The listing builds one solid part. Answer for the finished solid, in the listing's coordinates (mm). Coordinates: 2 decimals unless noted, no trailing zeros. Write each loop counter-clockwise with the first axis right and the second up, starting at its lowest first coordinate (ties: lowest second). Pieces come first, ordered by that corner, then holes. Notation, with made-up numbers: M 83,-12.5 L 112,-12.5 A24 ccw 112,0.5 Z; hole C -15,61 d8. An arc over 180 degrees is marked long. Answer as CSV lines item,"result".
```python
from build123d import *

# Parameters (mm, degrees)
SKETCH_1_R               = 9.5
SKETCH_1_R_2             = 4.25
EXTRUDE_1_DEPTH          = 7
CUT_EXTRUDE_1_DEPTH      = 16.149257408
CUT_EXTRUDE_1_DEPTH_BACK = 16.149257408
SKETCH_3_R               = 10
FILLET_1_R               = 1


with BuildPart() as part:
    # Эскиз1 → Бобышка-Вытянуть1 (new body)
    with BuildSketch(Plane.XY):
        Circle(SKETCH_1_R)
        Circle(SKETCH_1_R_2, mode=Mode.SUBTRACT)
    extrude(amount=EXTRUDE_1_DEPTH)

    # Эскиз3 → Вырез-Вытянуть1 (cut, two sides: drawn at the far end of the back side and taken through both)
    with BuildSketch(Plane(origin=(0, 0, 0), x_dir=(0, 0, -1), z_dir=(1, 0, 0)).offset(-CUT_EXTRUDE_1_DEPTH_BACK)):
        with Locations((6, 0.166135782)):
            Circle(SKETCH_3_R)
    extrude(amount=CUT_EXTRUDE_1_DEPTH + CUT_EXTRUDE_1_DEPTH_BACK, mode=Mode.SUBTRACT)

    # Скругление1
    fillet_1_edges = [part.edges().sort_by_distance(p)[0] for p in [
        (-9.5, 0, 7),
    ]]
    fillet(fillet_1_edges, radius=FILLET_1_R)


solid = part.part
```
Q1. Straight lines are drawn through the part: line 1 (Y direction, x = 0, z = 4.15); line 2 (Z direction, x = 1, y = 8.5). For each, find the intervals that lie inside material, in ascending order.
Output:
line 1,"-9.5 to -4.25, 4.25 to 9.5"
line 2,"0 to 7"
Q2. Find section D-D (z = 2.25). Give the vertices of the cut face in (x, y), and give its area (3 significant figures).
Output:
outline,"M -7.76,-5.49 A9.5 ccw 7.76,-5.49 Z; M -7.51,5.82 L 7.51,5.82 A9.5 ccw Z"
area,"82.3 mm2"
Q3. Flat-ended cylindrical pins translate along their axes: pin 1 Ø3 at (x, z) = (7.5, 6) entering from +Y; pin 2 Ø1 at (y, z) = (1.5, 5) entering from +X. Find the tip coordinate at first contact, or state that the pin passes through.
Output:
pin 1,"y = 7.37"
pin 2,"x = 9.45"
Q4. The mould has two halves that part along Y. Classify faces 1 (the cylindrical face through (4.38, -8.43, 3.62)), 2 (the cylindrical face through (-3.37, -2.59, 5.41)), 3 (the flat face through (-4, -2, 7)), 4 (the cylindrical face through (1.98, 4.29, 3.11)): pulls with the +Y half, pulls with the -Y half, needs draft (parallel to the pull), parting line crosses it, or undercut.
Output:
face 1,"parting line crosses it"
face 2,"undercut"
face 3,"needs draft"
face 4,"undercut"
Q5. Find section C-C (z = 0.75). Give the vertices of the cut face in (x, y).
Output:
outline,"M -6.18,-7.21 A9.5 ccw 6.18,-7.21 Z; M -5.77,7.54 L 5.77,7.54 A9.5 ccw Z"
Q6. Find section B-B (x = 0). Give the vertices of the cut face in (y, z).
Output:
outline,"M -9.5,0 L -7.83,0 A10 cw -4.25,2.97 L -4.25,7 L -8.5,7 A1 ccw -9.5,6 Z; M 4.25,3.13 A10 cw 8.17,0 L 9.5,0 L 9.5,6 A1 ccw 8.5,7 L 4.25,7 Z"
Q7. Find section A-A (y = 0). Give the vertices of the cut face in (x, z).
Output:
outline,"M -9.5,4 L -4.25,4 L -4.25,7 L -8.5,7 A1 ccw -9.5,6 Z; M 4.25,4 L 9.5,4 L 9.5,6 A1 ccw 8.5,7 L 4.25,7 Z"
